from build123d import *

# Parameters (mm, degrees)
BOSS_EXTRUDE1_DEPTH = 4
CUT_EXTRUDE1_DEPTH  = 10
FILLET1_R           = 2
FILLET2_R           = 2


with BuildPart() as part:
    # Sketch1 → Boss-Extrude1 (new body)
    with BuildSketch(Plane.XY):
        with BuildLine():
            Line((75.796342278, 15), (75.796342278, -15))
            Line((75.796342278, -15), (65.796342278, -15))
            Line((65.796342278, -15), (65.796342278, -10))
            Line((65.796342278, -10), (70.796342278, -10))
            Line((70.796342278, -10), (70.796342278, 0))
            Line((70.796342278, 0), (27.823693309, 0))
            Line((27.823693309, 0), (27.823693309, -5))
            Line((27.823693309, -5), (27.489306606, -5))
            ThreePointArc((27.489306606, -5), (24.977639534, -15), (27.489306606, -25))
            Line((27.489306606, -25), (2.888005027, -25))
            Line((2.888005027, -25), (2.888005027, -2))
            Line((2.888005027, -2), (-37.176306691, -2))
            Line((-37.176306691, -2), (-37.176306691, 25))
            Line((-37.176306691, 25), (-12.176306691, 25))
            Line((-12.176306691, 25), (-12.176306691, 15))
            Line((-12.176306691, 15), (75.796342278, 15))
        make_face()
    extrude(amount=BOSS_EXTRUDE1_DEPTH)

    # Sketch2 → Cut-Extrude1 (cut)
    with BuildSketch(Plane.XY.offset(4)):
        Polygon((-37.176306691, 19), (-32.133784184, 25), (-32.133784184, 30.908724767), (-39.468083963, 30.908724767), (-39.468083963, -2.242682287), (-33.176306691, -2.242682287), (-33.176306691, 2), (-37.176306691, 3), (-33.176306691, 10), (-37.176306691, 11), (-33.176306691, 18), align=None)
    extrude(amount=-CUT_EXTRUDE1_DEPTH, mode=Mode.SUBTRACT)

    # Fillet1
    fillet1_edges = [part.edges().sort_by_distance(p)[0] for p in [
        (65.796342278, -15, 2),
        (65.796342278, -10, 2),
        (70.796342278, -10, 2),
        (27.489306606, -25, 2),
    ]]
    fillet(fillet1_edges, radius=FILLET1_R)

    # Fillet2
    fillet2_edges = [part.edges().sort_by_distance(p)[0] for p in [
        (75.796342278, 15, 2),
        (70.796342278, 0, 2),
        (27.823693309, 0, 2),
        (-12.176306691, 15, 2),
    ]]
    fillet(fillet2_edges, radius=FILLET2_R)


solid = part.part
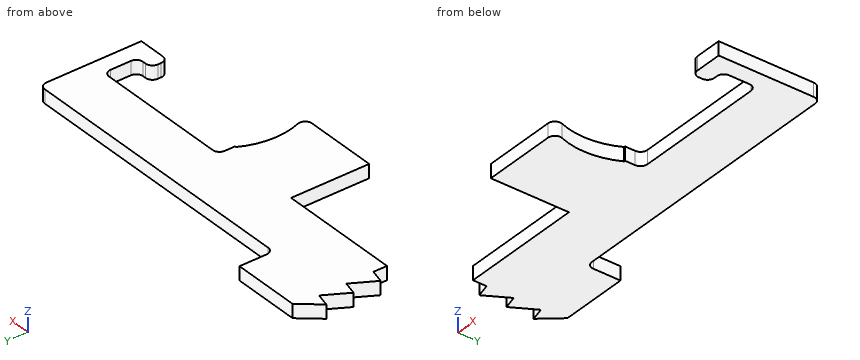
CAD build for the part. Positions are in the model's coordinates, mm. Coordinates: 2 decimals unless noted, no trailing zeros. Loops run counter-clockwise (first coordinate to the right, second up) from the corner with the lowest first, then second, coordinate; pieces in that order, holes last. Notation, with made-up numbers: (87, -17.75) -> (103, -17.75) arc R22 cw to (103, 8.25) -> close; hole circle Ø5 at (-24.5, 85). An arc over 180 degrees is marked (long way). One line per item, written item: value.
1. Drill centre lines: line 1 (Y direction, x = 42.5, z = 1.9); line 2 (Y direction, x = -22, z = 1.65); line 3 (X direction, y = -12.5, z = 3.5). Where is each one in solid material? Low to high. Write a range as [from, to].
Answers:
line 1: y = [0, 15]
line 2: y = [-2, 25]
line 3: x = [2.89, 25.13], [65.8, 75.8]
2. Slice it at A-A on x = -13.5. Write the cut outline in (y, z).
Answers:
outline: (-2, 0) -> (25, 0) -> (25, 4) -> (-2, 4) -> close
3. Slice it at C-C on y = 1. Write the cut outline in (x, z).
Answers:
outline: (-33.18, 0) -> (75.8, 0) -> (75.8, 4) -> (-33.18, 4) -> close
4. Flat gauge pins, fed straight in: P1, Ø2, axis at y = -5, z = 3, coming from the -X side; P2, Ø1.2, axis at y = -0.5, z = 1.5, coming from the -X side; P3, Ø2, axis at x = -13, z = 2, coming from the -Y side. Where does each tip first touch, or does it go through?
Answers:
P1: stops at x = 2.89
P2: stops at x = -33.18
P3: stops at y = -2
